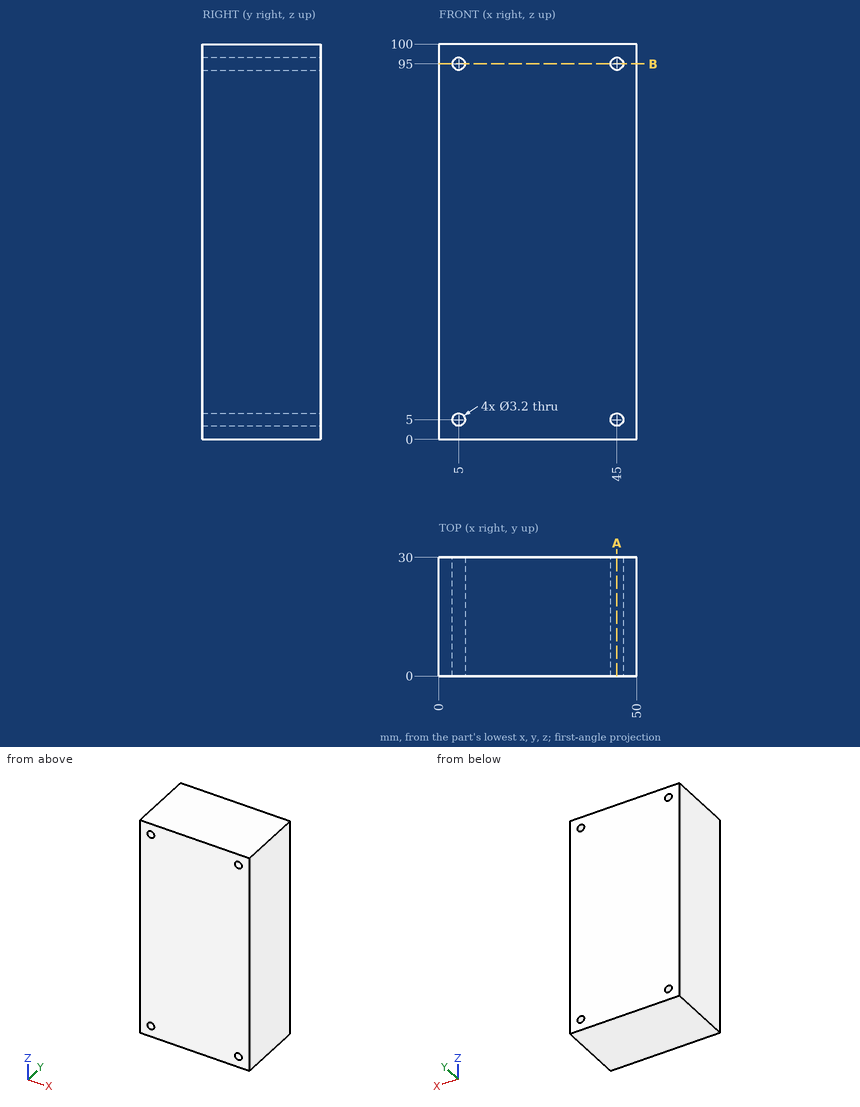
Answer from the drawing. Dimensions are ordinates in mm from the lowest x, y and z of the part. Coordinates: 2 decimals unless noted, no trailing zeros. Write each loop counter-clockwise with the first axis right and the second up, starting at its lowest first coordinate (ties: lowest second). Pieces come first, ordered by that corner, then holes. Notation, with made-up numbers: (71.5, 46) - (107.5, 46) arc R22 cw to (107.5, 83) - close; hole circle Ø8 at (86.5, 5.5). An arc over 180 degrees is marked (long way). Return JSON: item names as keys, results as strings. Group by question number.
Q1. The part is cut by section A-A on x = 45. Write down the section's boundary in (y, z).
Q2. Find the intervals of material crossed by line 1 along X through (y, z) = (19.25, 5); line 2 along Z through (x, y) = (5, 11.25), in increasing order. Write a range as [from, to].
Q3. A flat-ended cylindrical pin translates along its axis: pin 1 Ø1.9 at (x, z) = (5, 5) entering from +Y. Find the tip coordinate at first contact, or state that the pin passes through.
Q4. The part is cut by section B-B on z = 95. Write down the section's boundary in (x, y).
Evaluation:
{
 "1": {"outline": "(0, 0) - (30, 0) - (30, 3.4) - (0, 3.4) - close; (0, 6.6) - (30, 6.6) - (30, 93.4) - (0, 93.4) - close; (0, 96.6) - (30, 96.6) - (30, 100) - (0, 100) - close"},
 "2": {"line 1": "x = [0, 3.4], [6.6, 43.4], [46.6, 50]", "line 2": "z = [0, 3.4], [6.6, 93.4], [96.6, 100]"},
 "3": {"pin 1": "passes through"},
 "4": {"outline": "(0, 0) - (3.4, 0) - (3.4, 30) - (0, 30) - close; (6.6, 0) - (43.4, 0) - (43.4, 30) - (6.6, 30) - close; (46.6, 0) - (50, 0) - (50, 30) - (46.6, 30) - close"}
}
